```python
from build123d import *

# Parameters (mm, degrees)
F1_DEPTH = 12.7
F2_R     = 6.35
F3_DEPTH = 25.4


with BuildPart() as f1:
    # F0 (on Front) → F1 (new body)
    with BuildSketch(Plane.XZ):
        with BuildLine():
            ThreePointArc((8.798818, 10.16), (0, 15.24), (-8.798818, 10.16))
            Line((-8.798818, 10.16), (-35.651182, -36.349658))
            ThreePointArc((-35.651182, -36.349658), (-35.651182, -46.509658), (-26.852364, -51.589658))
            Line((-26.852364, -51.589658), (26.852364, -51.589658))
            ThreePointArc((26.852364, -51.589658), (35.651182, -46.509658), (35.651182, -36.349658))
            Line((35.651182, -36.349658), (8.798818, 10.16))
        make_face()
    extrude(amount=F1_DEPTH)

    # F2 (on face) → F3 (cut)
    with BuildSketch(Plane.XZ.offset(12.7)):
        with Locations((0, -25.926439)):
            Circle(F2_R)
    extrude(amount=-F3_DEPTH, mode=Mode.SUBTRACT)


solid = f1.part
```
The listing builds one solid part. Answer for the finished solid, in the listing's coordinates (mm). Give positions to 0.01 mm unless a question says otherwise; leave off trailing zeros. Write each loop counter-clockwise with the first axis right and the second up, starting at its lowest first coordinate (ties: lowest second). Pieces come first, ordered by that corner, then holes. Notation, with made-up numbers: (70, 7.5) -> (125, 7.5) arc R18 cw to (125, 29.5) -> close; hole circle Ø8 at (33, 44). An arc over 180 degrees is marked (long way). Write item = value, one per line. Start each with the question number.
1) The part is cut by section A-A, the plane x = 0. Determine the outline of the cut face in (y, z), and give its area (3 significant figures).
2) Straight lines are drawn through the part: line 1 along X through (y, z) = (-2.75, -28); line 2 along X through (y, z) = (-4, -24.5); line 3 along X through (y, z) = (-4.5, -40.5). For each, find the intervals that lie inside material, in ascending order.
3) Determine the mould class of faces 1 (the face through (0, -6, -51.59)), 2 (the face through (22.4, -6.3, -13.4)), 3 (the face through (-1.377, -6.439, -32.125)), 4 (the face through (-22.037, -6.261, -12.769)) for opening direction X: +X half, -X half, draft (parallel to the pull), parting line (faces both ways), or undercut.
4) Each of these flat-tipped pins is pushed along its axis until it touches: pin 1 (6 mm diameter, centred on y = -3.5, z = -3.5, fed in from -X); pin 2 (1.5 mm diameter, centred on y = -6, z = 3, fed in from -X); pin 3 (1 mm diameter, centred on x = -9.5, y = -2, fed in from +Z). Where does it stop, or does it pass through?
5) The part is cut by section D-D, the plane x = 11.5. Determine the outline of the cut face in (y, z), and give its area (3 significant figures).
6) The part is cut by section B-B, the plane y = -6.25. Determine the outline of the cut face in (x, z).
7) The part is cut by section C-C, the plane z = -22. Determine the outline of the cut face in (x, y).
Solutions:
q1.outline = (-12.7, -51.59) -> (0, -51.59) -> (0, -32.28) -> (-12.7, -32.28) -> close; (-12.7, -19.58) -> (0, -19.58) -> (0, 15.24) -> (-12.7, 15.24) -> close
q1.area = 687 mm²
q2.line_1 = -30.83 to -6, 6 to 30.83
q2.line_2 = -28.81 to -6.19, 6.19 to 28.81
q2.line_3 = -36.97 to 36.97
q3.face_1 = draft
q3.face_2 = +X half
q3.face_3 = undercut
q3.face_4 = -X half
q4.pin_1 = -18.42
q4.pin_2 = -13.37
q4.pin_3 = 9.81
q5.outline = (-12.7, -51.59) -> (0, -51.59) -> (0, 5.48) -> (-12.7, 5.48) -> close
q5.area = 725 mm²
q6.outline = (-35.65, -36.35) arc R10.16 ccw to (-26.85, -51.59) -> (26.85, -51.59) arc R10.16 ccw to (35.65, -36.35) -> (8.8, 10.16) arc R10.16 ccw to (-8.8, 10.16) -> close; hole circle Ø12.7 at (0, -25.93)
q7.outline = (-27.37, -12.7) -> (-4.99, -12.7) -> (-4.99, 0) -> (-27.37, 0) -> close; (4.99, -12.7) -> (27.37, -12.7) -> (27.37, 0) -> (4.99, 0) -> close
